from build123d import *

# Parameters (mm, degrees)
F0_W     = 19
F0_H     = 19
F1_DEPTH = 25
F3_SIZE  = 2
F4_SIZE  = 2
F5_SIZE  = 2
F2_R     = 4
F6_DEPTH = 25


with BuildPart() as f1:
    # F0 (on Front) → F1 (new body)
    with BuildSketch(Plane.XZ):
        Rectangle(F0_W, F0_H)
    extrude(amount=F1_DEPTH)

    # F3
    f3_edges = [f1.edges().sort_by_distance(p)[0] for p in [
        (9.5, -12.5, -9.5),
        (9.5, -12.5, 9.5),
    ]]
    chamfer(f3_edges, length=F3_SIZE)

    # F4
    f4_edges = [f1.edges().sort_by_distance(p)[0] for p in [
        (-9.5, -12.5, 9.5),
    ]]
    chamfer(f4_edges, length=F4_SIZE)

    # F5
    f5_edges = [f1.edges().sort_by_distance(p)[0] for p in [
        (-9.5, -12.5, -9.5),
    ]]
    chamfer(f5_edges, length=F5_SIZE)

    # F2 (on face) → F6 (cut)
    with BuildSketch(Plane(origin=(0, 0, 0), x_dir=(-1, 0, 0), z_dir=(0, 1, 0))):
        Circle(F2_R)
    extrude(amount=-F6_DEPTH, mode=Mode.SUBTRACT)


solid = f1.part
Input: part model. Units: mm. Frame: model coordinates. Coordinates: 2 decimals unless noted, no trailing zeros. Loops run counter-clockwise (first coordinate to the right, second up) from the corner with the lowest first, then second, coordinate; pieces in that order, holes last. Notation, with made-up numbers: (87.25, 6.5) -> (144.25, 6.5) arc R12 cw to (144.25, 15.5) -> close; hole circle Ø6 at (-27.75, 74). An arc over 180 degrees is marked (long way). Write item = value, one per line. Start each with the question number.
Item 1: Mould query, pull axis X, two halves, no side actions, for faces 1 (the face through (-4.4, -25, 0.1)), 2 (the face through (0.867, -12.325, -3.905)), 3 (the face through (-9.5, -12, 0)), 4 (the face through (9, -12, -8)). Classes: pulls with the +X half, pulls with the -X half, needs draft (parallel to the pull), parting line crosses it, or undercut.
Item 2: Cut plane B-B, the plane x = 0. Return loops of the section in (y, z).
Item 3: Cut plane A-A, the plane z = 0. Return loops of the section in (x, y), plus the area to 3 significant figures.
Item 4: Material intervals for line 1 (Z direction, x = 0, y = -17); line 2 (X direction, y = -0.75, z = -3); line 3 (Z direction, x = -1.75, y = -3.5), sorted ascending.
Item 5: Cut plane C-C, the plane y = -13. Return loops of the section in (x, z).
Item 6: First-contact query: P1, Ø8, axis at x = 7.5, z = 3, coming from the +Y side. Flat tip, straight axial feed; report the tip coordinate or a pass-through.
Ans:
q1.face_1 = needs draft
q1.face_2 = undercut
q1.face_3 = pulls with the -X half
q1.face_4 = pulls with the +X half
q2.outline = (-25, -9.5) -> (0, -9.5) -> (0, -4) -> (-25, -4) -> close; (-25, 4) -> (0, 4) -> (0, 9.5) -> (-25, 9.5) -> close
q3.outline = (-9.5, -25) -> (-4, -25) -> (-4, 0) -> (-9.5, 0) -> close; (4, -25) -> (9.5, -25) -> (9.5, 0) -> (4, 0) -> close
q3.area = 275 mm²
q4.line_1 = -9.5 to -4, 4 to 9.5
q4.line_2 = -9.5 to -2.65, 2.65 to 9.5
q4.line_3 = -9.5 to -3.6, 3.6 to 9.5
q5.outline = (-9.5, -7.5) -> (-7.5, -9.5) -> (7.5, -9.5) -> (9.5, -7.5) -> (9.5, 7.5) -> (7.5, 9.5) -> (-7.5, 9.5) -> (-9.5, 7.5) -> close; hole circle Ø8 at (0, 0)
q6.P1 = 0
